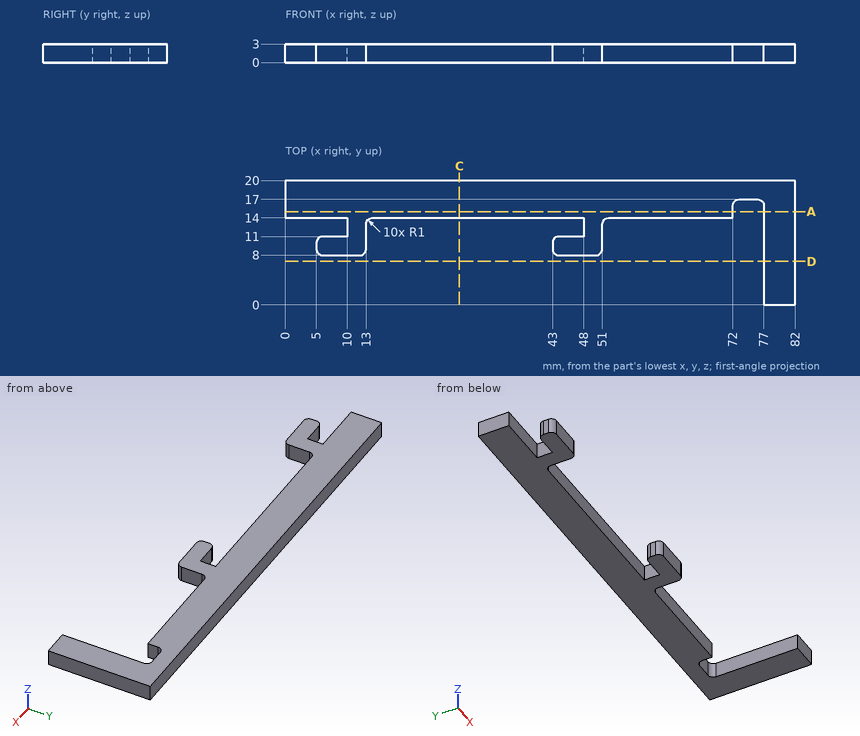
The drawing under review shows one solid part. Ordinate dimensions are in mm from its lowest x, y, z. Round coordinates to 2 decimals unless told otherwise and drop trailing zeros. Write each loop counter-clockwise with the first axis right and the second up, starting at its lowest first coordinate (ties: lowest second). Pieces come first, ordered by that corner, then holes. Notation, with made-up numbers: (45, 84) -> (70, 84) arc R21 cw to (70, 109) -> close; hole circle Ø11 at (-28, 22). An arc over 180 degrees is marked (long way). Put each result on its own line as item: value.
Q1. To check wall thickness, follow L1, parallel to X at y = 11.25, z = 1.1; L2, parallel to Y at x = 44.5, z = 2.4; L3, parallel to X at y = 14.25, z = 0.2. State the ranges of each line that lie inside material, in increasing order. Write a range as [from, to].
Determined:
L1: x = [10, 13], [48, 51], [77, 82]
L2: y = [8, 11], [14, 20]
L3: x = [0, 72], [77, 82]
Q2. Clearance check with flat-ended pins moving along their axes: pin 1 Ø0.9 at (x, z) = (67, 1) entering from -Y; pin 2 Ø0.9 at (y, z) = (12, 2) entering from -X; pin 3 Ø1.5 at (x, z) = (46.5, 2.5) entering from -Y. State where each tip first meets the part, or that it passes through.
Determined:
pin 1: stops at y = 14
pin 2: stops at x = 10
pin 3: stops at y = 8
Q3. Consider section D-D on y = 7. State the section outline as (x, z) points.
Determined:
outline: (77, 0) -> (82, 0) -> (82, 3) -> (77, 3) -> close
Q4. Consider section C-C on x = 28. State the section outline as (y, z) points, and give its area (3 significant figures).
Determined:
outline: (14, 0) -> (20, 0) -> (20, 3) -> (14, 3) -> close
area: 18.0 mm^2
Q5. Consider section A-A on y = 15. State the section outline as (x, z) points.
Determined:
outline: (0, 0) -> (72, 0) -> (72, 3) -> (0, 3) -> close; (77, 0) -> (82, 0) -> (82, 3) -> (77, 3) -> close
